Autodesk Inventor part; units mm, degrees
ref_plane "YZ Plane" through (0, 0, 0) normal (1, 0, 0) x (0, 1, 0)
ref_plane "XZ Plane" through (0, 0, 0) normal (0, 1, 0) x (-1, 0, 0)
ref_plane "XY Plane" through (0, 0, 0) normal (0, 0, 1) x (1, 0, 0)
sketch "Эскиз1" plane through (0, 0, 0) normal (0, 1, 0) x (-1, 0, 0)
  line L0 (11.5, 0) -> (-11.5, 0) construction
  line L1 (11.5, 2.5) -> (-11.5, 2.5)
  line L2 (-11.5, -2.5) -> (11.5, -2.5)
  arc A0 (11.5, -2.5) -> (11.5, 2.5) centre (11.5, 0) ccw
  arc A1 (-11.5, 2.5) -> (-11.5, -2.5) centre (-11.5, 0) ccw
  circle A2 centre (11.5, 0) radius 1.325
  circle A3 centre (-11.5, 0) radius 1.325
  line L3 (16.5, 7.5) -> (-6.5, 7.5)
  line L4 (-6.5, 2.5) -> (16.5, 2.5)
  arc A4 (16.5, 2.5) -> (16.5, 7.5) centre (16.5, 5) ccw
  arc A5 (-6.5, 7.5) -> (-6.5, 2.5) centre (-6.5, 5) ccw
  line L5 (11.5, 0) -> (16.5, 5) construction
  point P0 (0, 0)
  point P1 (0, 0)
  point P2 (-14, 0)
  point P3 (14, 0)
  point P4 (-9, 5)
  point P5 (19, 5)
  dimension "d0" = 2.65
  dimension "d1" = 2.65
  dimension "d2" = 2.5
  dimension "d6" = 2.5
  dimension "d12" = 45
  dimension "d16" = 23
  dimension "d28" = 5
  dimension "d29" = 7.0711
extrude "Выдавливание1" add sketch "Эскиз1" along normal blind 1.75 contours A0 L2 A1 L1
pattern_linear "Прямоуг.массив1" count 2 spacing 7.55 along (0, 1, 0) of "Выдавливание1"
sketch "Эскиз2" plane through (0, 0, 0) normal (0, 0, 1) x (1, 0, 0)
  arc A0 (1.575, 6.1) -> (-1.575, 6.1) centre (0, 6.1) ccw
  line L0 (-11.5, 9.3) -> (11.5, 9.3)
  line L1 (-11.5, 0) -> (11.5, 0)
  line L2 (-1.575, 6.1) -> (-1.575, 0)
  line L3 (1.575, 6.1) -> (1.575, 0)
  line L4 (11.5, 7.55) -> (-11.5, 7.55)
  line L5 (-3.25, 7.55) -> (-3.25, 0)
  line L6 (3.25, 7.55) -> (3.25, 0)
  line L7 (0, -1.86) -> (0, 11.16) construction
  point P0 (0.6149, 7.55)
  point P1 (-0.6149, 7.55)
  dimension "d21" = 3.15
  dimension "d33" = 3.2
  dimension "d34" = 3.25
  dimension "d35" = 3.25
extrude "Выдавливание2" cut sketch "Эскиз2" along normal mid plane 5 contours L3 L1 L2 A0 L4 | L4 A0
extrude "Выдавливание3" add sketch "Эскиз2" along normal mid plane 5 contours A0 L4 L6 L1 L3 | A0 L2 L1 L5 L4
properties part number "Чертёж"
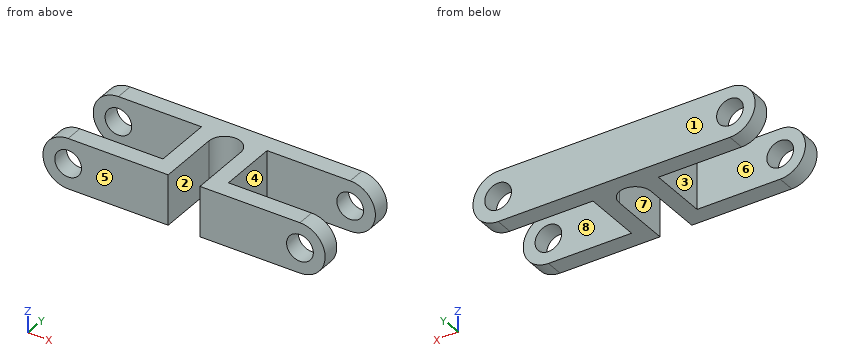
Work out the finished part from the listing and answer in its coordinate system (mm). Face numbers are marked on the shaded views. A direction names the side the tool comes from. Coordinates: 2 decimals unless noted, no trailing zeros. Loops run counter-clockwise (first coordinate to the right, second up) from the corner with the lowest first, then second, coordinate; pieces in that order, holes last.
1) For a pull along Y with two mould halves and no side action, classify the marked faces 5, 6, 7 and 8 as +Y half, -Y half, draft (parallel to the pull), parting line (faces both ways), or undercut.
Results:
face 5: -Y half
face 6: undercut
face 7: draft
face 8: undercut
2) Flat-ended cylindrical pins translate along their axes: pin 1 (5 mm diameter, centred on x = 0, y = 1.5, fed in from +Z); pin 2 (2.5 mm diameter, centred on y = 5.5, z = 1, fed in from +X); pin 3 (2 mm diameter, centred on x = 11.5, z = 0, fed in from -Y); pin 4 (2.5 mm diameter, centred on y = 3.5, z = 0.5, fed in from -X). Find the tip coordinate at first contact, or state that the pin passes through.
Results:
pin 1: stops at z = 2.5
pin 2: stops at x = 3.25
pin 3: passes through
pin 4: stops at x = -3.25
3) Section A-A (y = 2.5) is taken. Give the vertices of the cut face in (x, z) (3 decimals).
Results:
outline: (-3.25, -2.5) - (-1.575, -2.5) - (-1.575, 2.5) - (-3.25, 2.5) - close; (1.575, -2.5) - (3.25, -2.5) - (3.25, 2.5) - (1.575, 2.5) - close
4) Section D-D (x = 12.5) is taken. Give the vertices of the cut face in (y, z).
Results:
outline: (0, -2.29) - (1.75, -2.29) - (1.75, -0.87) - (0, -0.87) - close; (0, 0.87) - (1.75, 0.87) - (1.75, 2.29) - (0, 2.29) - close; (7.55, -2.29) - (9.3, -2.29) - (9.3, -0.87) - (7.55, -0.87) - close; (7.55, 0.87) - (9.3, 0.87) - (9.3, 2.29) - (7.55, 2.29) - close
5) Consider probe 1 along X at (y, z) = (8.5, -0.1); probe 2 along X at (y, z) = (5.5, 1.35) (3 decimals); probe 3 along Y at (x, z) = (-5.25, -1.55). Determine where each line is inside the solid, lowest interval first.
Results:
probe 1: x = -14 to -12.82, -10.18 to 10.18, 12.82 to 14
probe 2: x = -3.25 to -1.575, 1.575 to 3.25
probe 3: y = 0 to 1.75, 7.55 to 9.3
6) Section C-C (z = 0) is taken. Give the number of separate pieces and of enclosed holes in the cut face, plus the area to 3 significant figures.
Results:
separate pieces: 5
enclosed holes: 0
area: 94.0 mm2
7) Section B-B (x = -5.25) is taken. Give the vertices of the cut face in (y, z).
Results:
outline: (0, -2.5) - (1.75, -2.5) - (1.75, 2.5) - (0, 2.5) - close; (7.55, -2.5) - (9.3, -2.5) - (9.3, 2.5) - (7.55, 2.5) - close
8) For the marked faces 1, 2, 3 and 4, determine the directions among +Z, -Z, +X, -X, +Y, -Y from which every point of the face is accessible in a straight line to the end or side of a thin tool.
Results:
face 1: +Z, -Z, +X, -X, +Y
face 2: +Z, -Z, -Y
face 3: +Z, -Z, -X
face 4: +Z, -Z, +X
